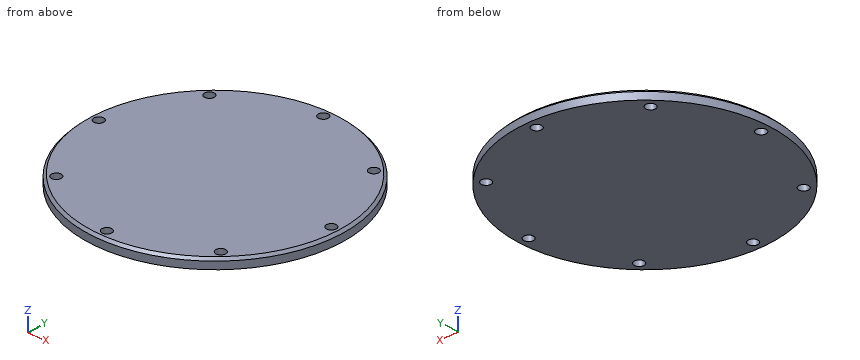
```python
from build123d import *

# Parameters (mm, degrees)
SKETCH_1_R          = 26
EXTRUDE_1_DEPTH     = 2
SKETCH_2_R          = 1
CUT_EXTRUDE_1_DEPTH = 2
CHAMFER_2_SIZE      = 0.5


with BuildPart() as part:
    # Эскиз1 → Бобышка-Вытянуть1 (new body)
    with BuildSketch(Plane.XY):
        Circle(SKETCH_1_R)
    extrude(amount=EXTRUDE_1_DEPTH)

    # Эскиз2 → Вырез-Вытянуть1 (cut)
    with BuildSketch(Plane.XY.offset(2)):
        with Locations((0, 24)):
            Circle(SKETCH_2_R)
        with Locations((16.970562748, 16.970562748)):
            Circle(SKETCH_2_R)
        with Locations((24, 0)):
            Circle(SKETCH_2_R)
        with Locations((16.970562748, -16.970562748)):
            Circle(SKETCH_2_R)
        with Locations((0, -24)):
            Circle(SKETCH_2_R)
        with Locations((-16.970562748, -16.970562748)):
            Circle(SKETCH_2_R)
        with Locations((-24, 0)):
            Circle(SKETCH_2_R)
        with Locations((-16.970562748, 16.970562748)):
            Circle(SKETCH_2_R)
    extrude(amount=-CUT_EXTRUDE_1_DEPTH, mode=Mode.SUBTRACT)

    # Фаска2
    chamfer_2_edges = [part.edges().sort_by_distance(p)[0] for p in [
        (-26, 0, 2),
    ]]
    chamfer(chamfer_2_edges, length=CHAMFER_2_SIZE)


solid = part.part
```
Geometry: final body of the model. Coordinates: model frame, mm. Round coordinates to 2 decimals unless told otherwise and drop trailing zeros. Write each loop counter-clockwise with the first axis right and the second up, starting at its lowest first coordinate (ties: lowest second). Pieces come first, ordered by that corner, then holes. Notation, with made-up numbers: M 54,9 L 102,9 A19 ccw 102,38 Z; hole C 76,40.25 d8. An arc over 180 degrees is marked long. Answer in a Markdown table with one row per item. Add a question column.
(1) Cut plane C-C, the plane z = 0.8. Give the number of separate pieces and of enclosed holes in the cut face, then the cut area to 3 significant figures.
(2) Ray query, L1, parallel to Y at x = 0, z = 0.6; L2, parallel to Y at x = -19, z = 1.5; L3, parallel to X at y = 5.5, z = 0.8. Return the intervals inside material, ascending.
(3) Contact query for flat-ended pins moving along their axis: pin 1 (1.8 mm diameter, centred on x = 16.97, y = 16.97, fed in from +Z); pin 2 (1 mm diameter, centred on x = 3, z = 0.5, fed in from -Y); pin 3 (1 mm diameter, centred on x = 6.5, z = 0.5, fed in from +Y); pin 4 (1 mm diameter, centred on y = -19, z = 1.5, fed in from +X). Output: stop coordinate, or through.
(4) Cut plane A-A, the plane y = 0. Return the cut outline in (x, z).
Established:
| question | item | result |
|---|---|---|
| 1 | separate pieces | 1 |
| 1 | enclosed holes | 8 |
| 1 | area | 2,100 mm² |
| 2 | L1 | -26 to -25, -23 to 23, 25 to 26 |
| 2 | L2 | -17.75 to 17.75 |
| 2 | L3 | -25.41 to 25.41 |
| 3 | pin 1 | through |
| 3 | pin 2 | y = -25.88 |
| 3 | pin 3 | y = 25.3 |
| 3 | pin 4 | x = 18.27 |
| 4 | outline | M -26,0 L -25,0 L -25,2 L -25.5,2 L -26,1.5 Z; M -23,0 L 23,0 L 23,2 L -23,2 Z; M 25,0 L 26,0 L 26,1.5 L 25.5,2 L 25,2 Z |
